```python
from build123d import *

# Parameters (mm, degrees)
SKETCH_1_W           = 20
SKETCH_1_H           = 20
EXTRUDE_1_DEPTH      = 4
SKETCH_2_W           = 12.9
SKETCH_2_H           = 20
EXTRUDE_2_DEPTH      = 3.8
SKETCH_3_R           = 1.6
CUT_EXTRUDE_1_DEPTH  = 30.340074983
SKETCH_4_W           = 5.8
SKETCH_4_H           = 20
SKETCH_4_R           = 1.6
EXTRUDE_3_DEPTH      = 1.5
SKETCH_5_R           = 3
CUT_EXTRUDE_3_DEPTH  = 2.4
SKETCH_6_W           = 20
SKETCH_6_H           = 4
EXTRUDE_4_DEPTH      = 3
EXTRUDE_START        = 4
SKETCH_7_W           = 23
SKETCH_7_H           = 20
SKETCH_7_R           = 3
EXTRUDE_5_DEPTH      = 4
SKETCH_9_W           = 10.1
SKETCH_9_H           = 20
EXTRUDE_6_DEPTH      = 2
EXTRUDE_7_DEPTH      = 5
CHAMFER_7_SIZE       = 10
CHAMFER_7_SIZE2      = 5.773502692
CHAMFER_8_SIZE       = 5
CHAMFER_9_SIZE       = 8
CHAMFER_9_SIZE2      = 4.618802154
CUT_EXTRUDE_9_DEPTH  = 10.1
CUT_EXTRUDE_10_REACH = 38.481
CHAMFER_10_SIZE      = 1.5
CHAMFER_11_SIZE      = 0.4


with BuildPart() as part:
    # 草图1 → 凸台-拉伸1 (new body)
    with BuildSketch(Plane(origin=(0, 0, 0), x_dir=(1, 0, 0), z_dir=(0, 1, 0))):
        with Locations((10, 10)):
            Rectangle(SKETCH_1_W, SKETCH_1_H)
    extrude(amount=EXTRUDE_1_DEPTH)

    # 草图2 → 凸台-拉伸2 (add)
    with BuildSketch(Plane(origin=(0, 4, 0), x_dir=(1, 0, 0), z_dir=(0, 1, 0))):
        with Locations((6.45, 10)):
            Rectangle(SKETCH_2_W, SKETCH_2_H)
    extrude(amount=EXTRUDE_2_DEPTH)

    # 草图3 → 切除-拉伸1 (cut, through all)
    with BuildSketch(Plane(origin=(0, 0, 0), x_dir=(-1, 0, 0), z_dir=(0, -1, 0))):
        with Locations(Location((-10, 5, 0), (0, 0, 90))):
            Circle(SKETCH_3_R)
        with Locations(Location((-10, 13, 0), (0, 0, 90))):
            Circle(SKETCH_3_R)
    extrude(amount=-CUT_EXTRUDE_1_DEPTH, mode=Mode.SUBTRACT)

    # 草图4 → 凸台-拉伸3 (add)
    with BuildSketch(Plane(origin=(0, 7.8, 0), x_dir=(1, 0, 0), z_dir=(0, 1, 0))):
        with Locations((10, 10)):
            Rectangle(SKETCH_4_W, SKETCH_4_H)
        with Locations(Location((10, 13, 0), (0, 0, 90))):
            Circle(SKETCH_4_R, mode=Mode.SUBTRACT)
        with Locations(Location((10, 5, 0), (0, 0, 90))):
            Circle(SKETCH_4_R, mode=Mode.SUBTRACT)
    extrude(amount=EXTRUDE_3_DEPTH)

    # 草图5 → 切除-拉伸3 (cut)
    with BuildSketch(Plane(origin=(0, 0, 0), x_dir=(-1, 0, 0), z_dir=(0, -1, 0))):
        with Locations(Location((-10, 5, 0), (0, 0, 90))):
            Circle(SKETCH_5_R)
        with Locations(Location((-10, 13, 0), (0, 0, 90))):
            Circle(SKETCH_5_R)
    extrude(amount=-CUT_EXTRUDE_3_DEPTH, mode=Mode.SUBTRACT)

    # 草图6 → 凸台-拉伸4 (add)
    with BuildSketch(Plane(origin=(20, 0, 0), x_dir=(0, 0, -1), z_dir=(1, 0, 0))):
        with Locations((10, 2)):
            Rectangle(SKETCH_6_W, SKETCH_6_H)
    extrude(amount=EXTRUDE_4_DEPTH)

    # 草图7 → 凸台-拉伸5 (add)
    with BuildSketch(Plane(origin=(0, 0, 0), x_dir=(-1, 0, 0), z_dir=(0, -1, 0)).offset(EXTRUDE_START)):
        with Locations((-11.5, 10)):
            Rectangle(SKETCH_7_W, SKETCH_7_H)
        with Locations(Location((-10, 13, 0), (0, 0, 90))):
            Circle(SKETCH_7_R, mode=Mode.SUBTRACT)
        with Locations(Location((-10, 5, 0), (0, 0, 90))):
            Circle(SKETCH_7_R, mode=Mode.SUBTRACT)
    extrude(amount=-EXTRUDE_5_DEPTH)

    # 草图9 → 凸台-拉伸6 (add)
    with BuildSketch(Plane(origin=(0, 4, 0), x_dir=(1, 0, 0), z_dir=(0, 1, 0))):
        with Locations((17.95, 10)):
            Rectangle(SKETCH_9_W, SKETCH_9_H)
    extrude(amount=EXTRUDE_6_DEPTH)

    # 草图11 → 凸台-拉伸7 (add)
    with BuildSketch(Plane(origin=(0, 0, -20), x_dir=(-1, 0, 0), z_dir=(0, 0, -1))):
        Polygon((-23, 6), (-23, -4), (0, -4), (0, 7.8), (-7.1, 7.8), (-7.1, 9.3), (-12.9, 9.3), (-12.9, 6), align=None)
    extrude(amount=EXTRUDE_7_DEPTH)

    # 倒角7
    chamfer_7_edges = [part.edges().sort_by_distance(p)[0] for p in [
        (0, -4, -12.5),
    ]]
    chamfer_7_side = [part.faces().sort_by_distance(p)[0] for p in [
        (0, 1.9, -12.5),
    ]]
    chamfer(chamfer_7_edges, length=CHAMFER_7_SIZE, length2=CHAMFER_7_SIZE2, reference=chamfer_7_side[0])

    # 倒角8
    chamfer_8_edges = [part.edges().sort_by_distance(p)[0] for p in [
        (23, 1, 0),
    ]]
    chamfer(chamfer_8_edges, length=CHAMFER_8_SIZE)

    # 倒角9
    chamfer_9_edges = [part.edges().sort_by_distance(p)[0] for p in [
        (20.5, -4, -2.5),
    ]]
    chamfer_9_side = [part.faces().sort_by_distance(p)[0] for p in [
        (20.5, 1, -2.5),
    ]]
    chamfer(chamfer_9_edges, length=CHAMFER_9_SIZE, length2=CHAMFER_9_SIZE2, reference=chamfer_9_side[0])

    # 草图15 → 切除-拉伸9 (cut)
    with BuildSketch(Plane(origin=(23, 0, 0), x_dir=(0, 0, -1), z_dir=(1, 0, 0))):
        Polygon((25, -3), (25, 6), (7, 6), align=None)
    extrude(amount=-CUT_EXTRUDE_9_DEPTH, mode=Mode.SUBTRACT)

    # 切除-拉伸10: up to this plane
    cut_extrude_10_end = Plane(origin=(-7.224611797, 6, -7), z_dir=(0, -0.894427190999916, 0.447213595499958))
    # 草图16 → 切除-拉伸10 (cut, up to the surface)
    with BuildSketch(Plane(origin=(0, 9.3, 0), x_dir=(1, 0, 0), z_dir=(0, 1, 0)), mode=Mode.PRIVATE) as cut_extrude_10_sk1:
        Polygon((7.9, 25), (12.9, 25), (12.9, 14), align=None)
    cut_extrude_10_tool1 = split(extrude(cut_extrude_10_sk1.sketch, amount=-CUT_EXTRUDE_10_REACH, mode=Mode.PRIVATE), bisect_by=cut_extrude_10_end, keep=Keep.BOTH, mode=Mode.PRIVATE)
    add(cut_extrude_10_tool1.solids().sort_by_distance((11.233333, 9.3, -21.333333))[0], mode=Mode.SUBTRACT)

    # 倒角10
    # the kernel refuses this chamfer: 1.5 mm, written as the material it takes off along each edge
    with BuildSketch(Plane(origin=(10, 2.4, -13), x_dir=(0, 0, -1), z_dir=(-1, 0, 0))) as chamfer_10_piece_1_section:
        Polygon((1.6, -CHAMFER_10_SIZE), (1.6 + CHAMFER_10_SIZE, 0), (1.6, 0), align=None)
    chamfer_10_piece_1 = revolve(axis=Axis((10, 2.4, -13), (0, -1, 0)), mode=Mode.PRIVATE)
    chamfer_10_piece_1 = chamfer_10_piece_1 & Plane(origin=(10, 2.4, -13), x_dir=(0, 0, -1), z_dir=(0, -1, 0)) * Cylinder(3, 13, mode=Mode.PRIVATE)
    add(chamfer_10_piece_1, mode=Mode.SUBTRACT)
    with BuildSketch(Plane(origin=(10, 2.4, -5), x_dir=(0, 0, -1), z_dir=(-1, 0, 0))) as chamfer_10_piece_2_section:
        Polygon((1.6, -CHAMFER_10_SIZE), (1.6 + CHAMFER_10_SIZE, 0), (1.6, 0), align=None)
    chamfer_10_piece_2 = revolve(axis=Axis((10, 2.4, -5), (0, -1, 0)), mode=Mode.PRIVATE)
    chamfer_10_piece_2 = chamfer_10_piece_2 & Plane(origin=(10, 2.4, -5), x_dir=(0, 0, -1), z_dir=(0, -1, 0)) * Cylinder(3, 13, mode=Mode.PRIVATE)
    add(chamfer_10_piece_2, mode=Mode.SUBTRACT)

    # 倒角11
    # the kernel refuses this chamfer: 0.4 mm, written as the material it takes off along each edge
    with BuildSketch(Plane(origin=(13.325667997, 9.3, -13.063530407), x_dir=(-0.9103664774626047, 4.440892098500618e-15, 0.41380294430118414), z_dir=(-0.4138029443011842, 0, -0.9103664774626047))) as chamfer_11_piece_1:
        Polygon((CHAMFER_11_SIZE, 0), (0, -CHAMFER_11_SIZE), (0, 0), align=None)
    extrude(amount=14.140392364, mode=Mode.SUBTRACT)
    with BuildSketch(Plane(origin=(12.9, 9.3, 1.028673195), x_dir=(-1, 0, 0), z_dir=(0, 0, -1))) as chamfer_11_piece_2:
        Polygon((CHAMFER_11_SIZE, 0), (0, -CHAMFER_11_SIZE), (0, 0), align=None)
    extrude(amount=16.05734639, mode=Mode.SUBTRACT)
    with BuildSketch(Plane(origin=(7.1, 9.3, 1.028673195), x_dir=(1, 0, 0), z_dir=(0, 0, -1))) as chamfer_11_piece_3:
        Polygon((CHAMFER_11_SIZE, 0), (0, CHAMFER_11_SIZE), (0, 0), align=None)
    extrude(amount=27.05734639, mode=Mode.SUBTRACT)


solid = part.part
```
CAD build for the part. Positions are in the model's coordinates, mm. A direction names the side the tool comes from. Round coordinates to 2 decimals unless told otherwise and drop trailing zeros. Loops run counter-clockwise (first coordinate to the right, second up) from the corner with the lowest first, then second, coordinate; pieces in that order, holes last. Notation, with made-up numbers: M 35.5,54 L 86.5,54 A25 cw 86.5,88 Z; hole C -24.75,63.5 d11. An arc over 180 degrees is marked long. Use a Markdown table: item, result. Add a question column.
(1) Cut at A-A (z = -13). Give the cut face in (x, y).
(2) Cut at C-C (x = 10). Give the cut face in (y, z), and give its area (3 significant figures).
(3) Pull direction X, two halves, no side cores. Call faces 5 (the face through (7.1, 8, -12)), 6 (the face through (9, 9.3, -10)), 7 (the face through (10.97, 6.56, -11.73)): +X half, -X half, draft (parallel to the pull), parting line (faces both ways), or undercut.
(4) Flat gauge pins, fed straight in: pin 1 (2 mm diameter, centred on x = 18, z = -4, fed in from +Y); pin 2 (3.5 mm diameter, centred on x = 4, z = -12, fed in from +Y); pin 3 (3.5 mm diameter, centred on x = 10, z = -5, fed in from -Y). Where does each tip first touch, or does it go through?
(5) Cut at D-D (z = -20). Give the cut face in (x, y).
(6) Drill centre lines: line 1 (Z direction, x = 10, y = 6.25); line 2 (Z direction, x = 8, y = -0.75); line 3 (X direction, y = 8.25, z = -5). Where is each one in solid material? Low to high.
(7) Which spindle directions (+Z, -Z, +X, -X, +Y, -Y) get a long thin tool onto all of the face, cutting with end or side? Do faces 1 (the face through (2.927, 0.93, -12.325)), 2 (the face through (10, -1, -10)), 3 (the face through (12.9, 7, -8)), 4 (the face through (17, 6, -3)). Say none if no direction does.
(8) Cut at B-B (y = 7). Give the cut face in (x, z).
Geometry says:
| question | item | result |
|---|---|---|
| 1 | outline | M 0,6 L 5.77,-4 L 7,-4 L 7,2.5 L 8.4,3.9 L 8.4,9.3 L 7.5,9.3 L 7.1,8.9 L 7.1,7.8 L 0,7.8 Z; M 11.6,3.9 L 13,2.5 L 13,-4 L 23,-4 L 23,3 L 12.9,3 L 12.9,8.9 L 12.5,9.3 L 11.6,9.3 Z |
| 2 | outline | M -4,-25 L -3,-25 L -0.69,-20.38 L 8.9,-20.38 L 9.3,-19.41 L 9.3,-14.6 L 3.9,-14.6 L 2.5,-16 L -4,-16 Z; M -4,-10 L 2.5,-10 L 3.9,-11.4 L 9.3,-11.4 L 9.3,-6.6 L 3.9,-6.6 L 2.5,-8 L -4,-8 Z; M -4,-2 L 2.5,-2 L 3.9,-3.4 L 9.3,-3.4 L 9.3,0 L -4,0 Z |
| 2 | area | 155 mm² |
| 3 | face 5 | -X half |
| 3 | face 6 | draft |
| 3 | face 7 | undercut |
| 4 | pin 1 | stops at y = 6 |
| 4 | pin 2 | stops at y = 7.8 |
| 4 | pin 3 | stops at y = 3.75 |
| 5 | outline | M 0,6 L 5.77,-4 L 23,-4 L 23,-0.5 L 10.17,-0.5 L 10.17,8.9 L 9.73,9.3 L 7.5,9.3 L 7.1,8.9 L 7.1,7.8 L 0,7.8 Z |
| 6 | line 1 | z = -20.38 to -14.6, -11.4 to -6.6, -3.4 to 0 |
| 6 | line 2 | z = -24.78 to -15.24, -10.76 to -7.24, -2.76 to 0 |
| 6 | line 3 | x = 7.1 to 8.4, 11.6 to 12.9 |
| 7 | face 1 | +Z, -Z, -X, -Y |
| 7 | face 2 | -Y |
| 7 | face 3 | -Z, +X, +Y |
| 7 | face 4 | +Z, -Z, +X, +Y |
| 8 | outline | M 0,-25 L 7.9,-25 L 12.9,-14 L 12.9,0 L 0,0 Z; hole C 10,-13 d3.2; hole C 10,-5 d3.2 |
